Source: CAD feature listing. Evaluate the final solid. Frame: model axes, mm. Face numbers are marked on the shaded views. A direction names the side the tool comes from. Coordinates: 2 decimals unless noted, no trailing zeros. Order: outer loops, then holes, each group sorted by start corner. A loop starts at its lowest first (then second) coordinate and runs counter-clockwise, first axis right, second up. Notation, with made-up numbers: (74.5, 26.25) -> (98.5, 26.25) arc R24 cw to (98.5, 42.25) -> close; hole circle Ø1 at (-34, -10.75). An arc over 180 degrees is marked (long way). Write item = value, one per line. Start each with the question number.
Item 1: Section query C-C (x = 9.5). Output: boundary loops of the cut face in (y, z).
Item 2: Mould query, pull axis X, two halves, no side actions, for the marked faces 4, 5 and 6. Classes: released by +X, released by -X, zero draft, split by the parting line, or undercut.
Item 3: Set-up query: the marked faces 1, 2 and 3. Return all of +Z, -Z, +X, -X, +Y, -Y with unobstructed straight access to the full face (end or side cutting, diameter ignored); none if empty.
Item 4: Section query B-B (y = -6). Output: boundary loops of the cut face in (x, z).
Item 5: Contact query for flat-ended pins moving along their axis: pin 1 (6.5 mm diameter, centred on x = 15.56, y = 15.56, fed in from -Z); pin 2 (3 mm diameter, centred on y = 6.5, z = -1, fed in from -X); pin 3 (2 mm diameter, centred on x = 16, y = -15.5, fed in from +Z); pin 4 (3 mm diameter, centred on x = -22.5, y = 8.5, fed in from +Z). Output: stop coordinate, or through.
Item 6: Ray query, line 1 along Y through (x, z) = (0, -0.05); line 2 along X through (y, z) = (-17.5, -0.75); line 3 along X through (y, z) = (-17, 1.55). Return the intervals inside material, ascending. Write a range as [from, to].
Item 7: Section query D-D (y = -14). Count the separate pieces of the cut face and the enclosed holes in it, then the cut area to 3 significant figures.
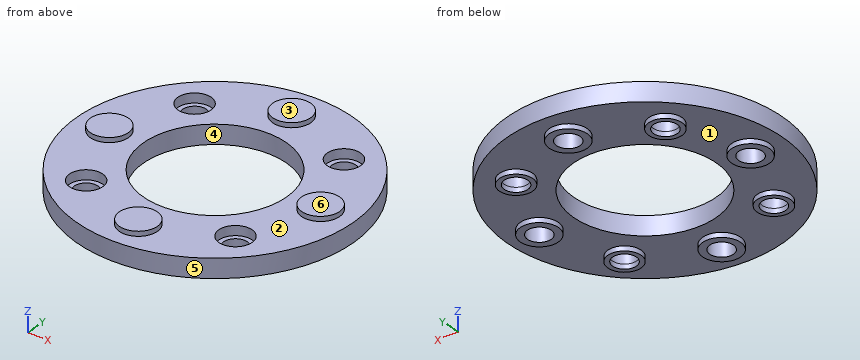
```python
from build123d import *

# Parameters (mm, degrees)
SKETCH_1_R                = 29.000000000000004
SKETCH_1_R_2              = 15.000000000000002
EXTRUDE_1_DEPTH           = 2
SKETCH_2_R                = 4.000000000000001
EXTRUDE_2_DEPTH           = 3
SKETCH_3_R                = 2.5
CUT_EXTRUDE_1_DEPTH       = 4.5
PATTERN_CIRCULAR_1_COUNT  = 4
HOLE_WIZARD_1_D           = 5
HOLE_WIZARD_1_CBORE_D     = 7
HOLE_WIZARD_1_CBORE_DEPTH = 2
SKETCH_6_R                = 3.5000000000000013
SKETCH_6_R_2              = 2.500000000000015
EXTRUDE_3_DEPTH           = 1
PATTERN_CIRCULAR_2_COUNT  = 4


with BuildPart() as part:
    # 草图1 → 凸台-拉伸1 (new, symmetric)
    with BuildSketch(Plane.XY):
        Circle(SKETCH_1_R)
        Circle(SKETCH_1_R_2, mode=Mode.SUBTRACT)
    extrude(amount=EXTRUDE_1_DEPTH, both=True)

    # 草图2 → 凸台-拉伸2 (add, symmetric)
    with BuildSketch(Plane.XY):
        with Locations((0, 22)):
            Circle(SKETCH_2_R)
    extrude_2 = extrude(amount=EXTRUDE_2_DEPTH, both=True)

    # 草图3 → 切除-拉伸1 (cut)
    with BuildSketch(Plane(origin=(0, 0, -3), x_dir=(-1, 0, 0), z_dir=(0, 0, -1))):
        with Locations((0, 22)):
            Circle(SKETCH_3_R)
    cut_extrude_1 = extrude(amount=-CUT_EXTRUDE_1_DEPTH, mode=Mode.SUBTRACT)

    # 阵列(圆周)1: 凸台-拉伸2, 切除-拉伸1 ×4 about axis
    pattern_circular_1_axis = Axis((-3.841e-14, 0, 0), (0, 0, 1))
    add([extrude_2.rotate(pattern_circular_1_axis, i * 360 / PATTERN_CIRCULAR_1_COUNT) for i in range(1, PATTERN_CIRCULAR_1_COUNT)])
    add([cut_extrude_1.rotate(pattern_circular_1_axis, i * 360 / PATTERN_CIRCULAR_1_COUNT) for i in range(1, PATTERN_CIRCULAR_1_COUNT)], mode=Mode.SUBTRACT)

    # 孔1 (through all)
    with Locations(Plane.XY.offset(2)):
        with Locations((-15.556349186, 15.556349186)):
            hole_wizard_1 = CounterBoreHole(HOLE_WIZARD_1_D / 2, HOLE_WIZARD_1_CBORE_D / 2, HOLE_WIZARD_1_CBORE_DEPTH)

    # 草图6 → 凸台-拉伸3 (add)
    with BuildSketch(Plane(origin=(0, 0, -2), x_dir=(-1, 0, 0), z_dir=(0, 0, -1))):
        with Locations(Location((15.556349186104072, 15.556349186104015, 0), (0, 0, 180))):
            Circle(SKETCH_6_R)
        with Locations(Location((15.556349186104072, 15.556349186104015, 0), (0, 0, 180))):
            Circle(SKETCH_6_R_2, mode=Mode.SUBTRACT)
    extrude_3 = extrude(amount=EXTRUDE_3_DEPTH)

    # 阵列(圆周)2: 孔1, 凸台-拉伸3 ×4 about axis
    pattern_circular_2_axis = Axis((2.732e-14, 2.732e-14, 0), (0, 0, 1))
    add([hole_wizard_1.rotate(pattern_circular_2_axis, i * 360 / PATTERN_CIRCULAR_2_COUNT) for i in range(1, PATTERN_CIRCULAR_2_COUNT)], mode=Mode.SUBTRACT)
    add([extrude_3.rotate(pattern_circular_2_axis, i * 360 / PATTERN_CIRCULAR_2_COUNT) for i in range(1, PATTERN_CIRCULAR_2_COUNT)])


solid = part.part
```
Computed:
q1.outline = (-27.4, -2) -> (-11.61, -2) -> (-11.61, 2) -> (-27.4, 2) -> close; (11.61, -2) -> (27.4, -2) -> (27.4, 2) -> (11.61, 2) -> close
q2.face_4 = undercut
q2.face_5 = split by the parting line
q2.face_6 = zero draft
q3.face_1 = -Z
q3.face_2 = +Z
q3.face_3 = +Z, +X, -X, +Y, -Y
q4.outline = (-28.37, -2) -> (-13.75, -2) -> (-13.75, 2) -> (-28.37, 2) -> close; (13.75, -2) -> (28.37, -2) -> (28.37, 2) -> (13.75, 2) -> close
q5.pin_1 = -3
q5.pin_2 = -28.57
q5.pin_3 = through
q5.pin_4 = 2
q6.line_1 = [-29, -24.5], [-19.5, -15], [15, 19.5], [24.5, 29]
q6.line_2 = [-23.12, -17.13], [-13.98, 13.98], [17.13, 23.12]
q6.line_3 = [-23.49, -18.74], [-12.37, 12.37], [18.74, 23.49]
q7.separate_pieces = 4
q7.enclosed_holes = 0
q7.area = 124 mm^2
